Work out the finished part from the listing and answer in its coordinate system (mm). Face numbers are marked on the shaded views. A direction names the side the tool comes from. Coordinates: 2 decimals unless noted, no trailing zeros. Write each loop counter-clockwise with the first axis right and the second up, starting at its lowest first coordinate (ties: lowest second). Pieces come first, ordered by that corner, then holes. Notation, with made-up numbers: M 36.25,-38 L 94.25,-38 A29 ccw 94.25,-9 Z; hole C 3.25,2 d7. An arc over 180 degrees is marked long. Answer as CSV lines item,"result". Start each with the question number.
(1) A cutting plane is placed at C-C on z = -3. Give the vertices of the cut face in (x, y) (3 decimals).
(2) Flat-ended cylindrical pins translate along their axes: P1, Ø0.5, axis at x = 113.5, y = -3, coming from the -Z side; P2, Ø0.5, axis at x = 114, y = -2.5, coming from the +Z side; P3, Ø1.1, axis at x = 114, y = -2.5, coming from the +Z side. Find the tip coordinate at first contact, or state that the pin passes through.
(3) Find the intervals of material crossed by L1, parallel to Z at x = 108.75, y = -8; L2, parallel to Z at x = 105.75, y = -3; L3, parallel to Z at x = 99.5, y = -10.5, in increasing order. Write a range as [from, to].
(4) A cutting plane is placed at A-A on y = -2.5. Count the separate pieces of the cut face and the enclosed holes in it, then the cut area to 3 significant figures.
(5) A cutting plane is placed at B-B on y = -11. Give the vertices of the cut face in (x, z) (3 decimals), then the cut area to 3 significant figures.
(6) The mould has two halves that part along Z. Classify the marked faces 1, 2 and 3: released by +Z, released by -Z, zero draft, split by the parting line, or undercut.
(7) For the marked faces 4, 5 and 6, determine the directions among +Z, -Z, +X, -X, +Y, -Y from which every point of the face is accessible in a straight line to the end or side of a thin tool.
from build123d import *

# Parameters (mm, degrees)
BOSS_EXTRUDE1_DEPTH = 18
SKETCH2_R           = 0.925
CUT_EXTRUDE1_DEPTH  = 3
SKETCH4_W           = 42.475453112
SKETCH4_H           = 12
BOSS_EXTRUDE2_DEPTH = 1
SKETCH5_W           = 42.475453112
SKETCH5_H           = 12
BOSS_EXTRUDE3_DEPTH = 1
SKETCH6_W           = 3
SKETCH6_H           = 3
SKETCH6_W_2         = 4
CUT_EXTRUDE2_DEPTH  = 48.044193641
FILLET1_R           = 1
FILLET2_R           = 1
SKETCH7_R           = 5
CUT_EXTRUDE3_DEPTH  = 1
SKETCH8_R           = 1
CUT_EXTRUDE4_DEPTH  = 1


with BuildPart() as part:
    # Sketch1 → Boss-Extrude1 (new body)
    with BuildSketch(Plane(origin=(95.165105206, 0, 0), x_dir=(0, 0, -1), z_dir=(1, 0, 0))):
        Polygon((34.286183253, -5.063386162), (16.286183253, -5.063386162), (16.286183253, -1.063386162), (-0.638816747, -1.063386162), (-0.638816747, -12.063386162), (-1.638816747, -12.063386162), (-1.638816747, -0.063386162), (0.242411468, -0.063386162), (19.150462688, -0.063386162), (40.836636365, -0.063386162), (40.836636365, -12.063386162), (39.036636365, -12.063386162), (39.036636365, -1.063386162), (17.286183253, -1.063386162), (17.286183253, -4.063386162), (35.286183253, -4.063386162), (35.286183253, -12.063386162), (34.286183253, -12.063386162), align=None)
    extrude(amount=BOSS_EXTRUDE1_DEPTH)

    # Sketch2 → Cut-Extrude1 (cut)
    with BuildSketch(Plane(origin=(0, 0, -40.836636365), x_dir=(-1, 0, 0), z_dir=(0, 0, -1))):
        with BuildLine():
            Line((-107.105470333, -6.019636162), (-105.000073019, -6.019636162))
            ThreePointArc((-105.000073019, -6.019636162), (-108.665105206, -3.063386162), (-112.330137394, -6.019636162))
            Line((-112.330137394, -6.019636162), (-110.22474008, -6.019636162))
            ThreePointArc((-110.22474008, -6.019636162), (-108.665105206, -5.063386162), (-107.105470333, -6.019636162))
        make_face()
        with BuildLine():
            ThreePointArc((-110.22474008, -7.607136162), (-108.665105206, -8.563386162), (-107.105470333, -7.607136162))
            Line((-107.105470333, -7.607136162), (-105.000073019, -7.607136162))
            ThreePointArc((-105.000073019, -7.607136162), (-108.665105206, -10.563386162), (-112.330137394, -7.607136162))
            Line((-112.330137394, -7.607136162), (-110.22474008, -7.607136162))
        make_face()
        with Locations((-108.665105206, -6.813386162)):
            Circle(SKETCH2_R)
        with Locations((-99.665105206, -6.813386162)):
            Circle(SKETCH2_R)
        with BuildLine():
            Line((-98.105470333, -6.019636162), (-96.000073019, -6.019636162))
            ThreePointArc((-96.000073019, -6.019636162), (-99.665105206, -3.063386162), (-103.330137394, -6.019636162))
            Line((-103.330137394, -6.019636162), (-101.22474008, -6.019636162))
            ThreePointArc((-101.22474008, -6.019636162), (-99.665105206, -5.063386162), (-98.105470333, -6.019636162))
        make_face()
        with BuildLine():
            Line((-101.22474008, -7.607136162), (-103.330137394, -7.607136162))
            ThreePointArc((-103.330137394, -7.607136162), (-99.665105206, -10.563386162), (-96.000073019, -7.607136162))
            Line((-96.000073019, -7.607136162), (-98.105470333, -7.607136162))
            ThreePointArc((-98.105470333, -7.607136162), (-99.665105206, -8.563386162), (-101.22474008, -7.607136162))
        make_face()
    extrude(amount=-CUT_EXTRUDE1_DEPTH, mode=Mode.SUBTRACT)

    # Sketch4 → Boss-Extrude2 (add)
    with BuildSketch(Plane(origin=(113.165105206, 0, 0), x_dir=(0, 0, -1), z_dir=(1, 0, 0))):
        with Locations((19.598909809, -6.063386162)):
            Rectangle(SKETCH4_W, SKETCH4_H)
    extrude(amount=BOSS_EXTRUDE2_DEPTH)

    # Sketch5 → Boss-Extrude3 (add)
    with BuildSketch(Plane.ZY.offset(-95.165105206)):
        with Locations((-19.598909809, -6.063386162)):
            Rectangle(SKETCH5_W, SKETCH5_H)
    extrude(amount=BOSS_EXTRUDE3_DEPTH)

    # Sketch6 → Cut-Extrude2 (cut, through all)
    with BuildSketch(Plane.ZY.offset(-94.165105206)):
        with Locations((-18.786183253, -2.563386162)):
            Rectangle(SKETCH6_W, SKETCH6_H)
        with Locations((-23.286183253, -2.563386162)):
            Rectangle(SKETCH6_W_2, SKETCH6_H)
        with Locations((-29.286183253, -2.563386162)):
            Rectangle(SKETCH6_W_2, SKETCH6_H)
        with Locations((-33.786183253, -2.563386162)):
            Rectangle(SKETCH6_W, SKETCH6_H)
    extrude(amount=-CUT_EXTRUDE2_DEPTH, mode=Mode.SUBTRACT)

    # Fillet1
    fillet1_edges = [part.edges().sort_by_distance(p)[0] for p in [
        (113.665105206, -4.063386162, -20.286183253),
        (113.665105206, -1.063386162, -20.286183253),
        (94.665105206, -4.063386162, -20.286183253),
        (94.665105206, -1.063386162, -20.286183253),
        (113.665105206, -1.063386162, -21.286183253),
        (113.665105206, -4.063386162, -25.286183253),
        (113.665105206, -1.063386162, -25.286183253),
        (94.665105206, -1.063386162, -21.286183253),
        (94.665105206, -4.063386162, -25.286183253),
        (94.665105206, -1.063386162, -25.286183253),
        (113.665105206, -1.063386162, -27.286183253),
        (113.665105206, -4.063386162, -31.286183253),
        (113.665105206, -1.063386162, -31.286183253),
        (94.665105206, -1.063386162, -27.286183253),
        (94.665105206, -4.063386162, -31.286183253),
        (94.665105206, -1.063386162, -31.286183253),
        (113.665105206, -4.063386162, -35.286183253),
        (113.665105206, -1.063386162, -35.286183253),
        (113.665105206, -1.063386162, -32.286183253),
        (94.665105206, -4.063386162, -35.286183253),
        (94.665105206, -1.063386162, -35.286183253),
        (94.665105206, -1.063386162, -32.286183253),
        (104.165105206, -1.063386162, -17.286183253),
    ]]
    fillet(fillet1_edges, radius=FILLET1_R)

    # Fillet2
    fillet2_edges = [part.edges().sort_by_distance(p)[0] for p in [
        (114.165105206, -6.063386162, -40.836636365),
        (114.165105206, -0.063386162, -19.598909809),
        (114.165105206, -6.063386162, 1.638816747),
        (94.165105206, -6.063386162, -40.836636365),
        (94.165105206, -6.063386162, 1.638816747),
        (94.165105206, -0.063386162, -19.598909809),
        (104.165105206, -0.063386162, -40.836636365),
        (104.165105206, -0.063386162, 1.638816747),
    ]]
    fillet(fillet2_edges, radius=FILLET2_R - 0.0001)  # a hair under: the kernel refuses the full size

    # Sketch7 → Cut-Extrude3 (cut)
    with BuildSketch(Plane(origin=(0, -4.063386162, 0), x_dir=(1, 0, 0), z_dir=(0, 1, 0))):
        with Locations(Location((103.665105206, 26.786183253, 0), (0, 0, 270))):
            Circle(SKETCH7_R)
    extrude(amount=-CUT_EXTRUDE3_DEPTH, mode=Mode.SUBTRACT)

    # Sketch8 → Cut-Extrude4 (cut)
    with BuildSketch(Plane.XY.offset(1.638816747)):
        with Locations((98.165105206, -4.063386162)):
            Circle(SKETCH8_R)
        with Locations((102.165105206, -4.063386162)):
            Circle(SKETCH8_R)
        with Locations((106.165105206, -4.063386162)):
            Circle(SKETCH8_R)
        with Locations((110.165105206, -4.063386162)):
            Circle(SKETCH8_R)
    extrude(amount=-CUT_EXTRUDE4_DEPTH, mode=Mode.SUBTRACT)


solid = part.part
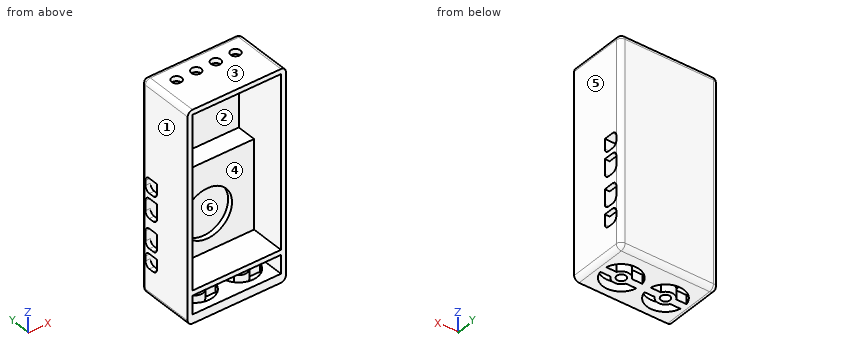
Here are the results:
1,outline,"M 94.165,-12.063 L 95.165,-12.063 L 95.165,-1.063 L 113.165,-1.063 L 113.165,-12.063 L 114.165,-12.063 L 114.165,-1.063 A1 ccw 113.165,-0.063 L 95.165,-0.063 A1 ccw 94.165,-1.063 Z"
2,P1,"stops at z = -40.83"
2,P2,"stops at z = 1.45"
2,P3,"stops at z = 1.6"
3,L1,"z = [-40.84, -39.04], [-35.29, -34.29], [0.64, 1.64]"
3,L2,"z = [-40.84, -39.04], [-17.29, -16.29], [0.64, 1.64]"
3,L3,"z = [-35.29, -34.29], [0.64, 1.64]"
4,separate pieces,"8"
4,enclosed holes,"1"
4,area,"124 mm^2"
5,outline,"M 94.165,-39.837 A1 ccw 95.165,-40.837 L 113.165,-40.837 A1 ccw 114.165,-39.837 L 114.165,0.639 A1 ccw 113.165,1.639 L 95.165,1.639 A1 ccw 94.165,0.639 Z; hole M 95.165,-39.037 L 113.165,-39.037 L 113.165,-35.286 L 95.165,-35.286 Z; hole M 95.165,-34.286 L 113.165,-34.286 L 113.165,0.639 L 95.165,0.639 Z"
5,area,"152 mm^2"
6,face 1,"zero draft"
6,face 2,"undercut"
6,face 3,"released by +Z"
7,face 4,"-Y"
7,face 5,"+Z, -Z, +X, +Y, -Y"
7,face 6,"none"
